Design review of the part built by this model. Coordinates are the model's own, in mm. Face numbers are marked on the shaded views. A direction names the side the tool comes from. Give positions to 0.01 mm unless a question says otherwise; leave off trailing zeros. Write each loop counter-clockwise with the first axis right and the second up, starting at its lowest first coordinate (ties: lowest second). Pieces come first, ordered by that corner, then holes. Notation, with made-up numbers: M 48,61 L 102,61 A22 cw 102,96 Z; hole C 82.25,-6.75 d8. An arc over 180 degrees is marked long. Answer in a Markdown table with one row per item.
```python
from build123d import *

# Parameters (mm, degrees)
F1_DEPTH = 15
F3_DEPTH = 54.4625242271
F5_DEPTH = 54.4625242271
F7_DEPTH = 53.9625242271
F8_R     = 5


with BuildPart() as f1:
    # F0 (on Top) → F1 (new body)
    with BuildSketch(Plane.XY):
        with BuildLine():
            Line((-25.9807621135, 15), (-30.3108891325, 17.5))
            ThreePointArc((-30.3108891325, 17.5), (-30.7987090687, 16.6264704522), (-31.2613615027, 15.7393544021))
            ThreePointArc((-31.2613615027, 15.7393544021), (-30.057560378, -17.9316219045), (-1, -34.9857113691))
            Line((-1, -34.9857113691), (-1, -32.5))
            Line((-1, -32.5), (1, -32.5))
            Line((1, -32.5), (1, -34.9857113691))
            ThreePointArc((1, -34.9857113691), (30.057560378, -17.9316219045), (31.2613615027, 15.7393544021))
            ThreePointArc((31.2613615027, 15.7393544021), (30.7987090687, 16.6264704522), (30.3108891325, 17.5))
            Line((30.3108891325, 17.5), (25.9807621135, 15))
            ThreePointArc((25.9807621135, 15), (0, -30), (-25.9807621135, 15))
        make_face()
        with BuildLine():
            ThreePointArc((-31.2613615027, 15.7393544021), (-30.7987090687, 16.6264704522), (-30.3108891325, 17.5))
            Line((-30.3108891325, 17.5), (-51.9615242271, 30))
            Line((-51.9615242271, 30), (-52.9615242271, 28.2679491924))
            Line((-52.9615242271, 28.2679491924), (-31.2613615027, 15.7393544021))
        make_face()
        with BuildLine():
            Line((-1, -32.5), (-1, -34.9857113691))
            ThreePointArc((-1, -34.9857113691), (0, -35), (1, -34.9857113691))
            Line((1, -34.9857113691), (1, -32.5))
            Line((1, -32.5), (-1, -32.5))
        make_face()
        with BuildLine():
            ThreePointArc((1, -34.9857113691), (0, -35), (-1, -34.9857113691))
            Line((-1, -34.9857113691), (-1, -57.5))
            Line((-1, -57.5), (1, -57.5))
            Line((1, -57.5), (1, -34.9857113691))
        make_face()
        with BuildLine():
            Line((51.9615242271, 30), (30.3108891325, 17.5))
            ThreePointArc((30.3108891325, 17.5), (30.7987090687, 16.6264704522), (31.2613615027, 15.7393544021))
            Line((31.2613615027, 15.7393544021), (52.9615242271, 28.2679491924))
            Line((52.9615242271, 28.2679491924), (51.9615242271, 30))
        make_face()
    extrude(amount=F1_DEPTH)

    # F2 (on face) → F3 (cut, through all)
    with BuildSketch(Plane(origin=(-1, -1.7320508076, 0), x_dir=(0.8660254038, -0.5, 0), z_dir=(-0.5, -0.8660254038, 0))):
        with BuildLine():
            Line((-37.4714052097, 15), (-57.4714052097, 15))
            ThreePointArc((-57.4714052097, 15), (-47.4714052097, 5), (-37.4714052097, 15))
        make_face()
    extrude(amount=-F3_DEPTH, mode=Mode.SUBTRACT)

    # F4 (on face) → F5 (cut, through all)
    with BuildSketch(Plane(origin=(1, -1.7320508076, 0), x_dir=(0.8660254038, 0.5, 0), z_dir=(0.5, -0.8660254038, 0))):
        with BuildLine():
            Line((57.4714052097, 15), (37.4714052097, 15))
            ThreePointArc((37.4714052097, 15), (47.4714052097, 5), (57.4714052097, 15))
        make_face()
    extrude(amount=-F5_DEPTH, mode=Mode.SUBTRACT)

    # F6 (on face) → F7 (cut, through all)
    with BuildSketch(Plane.YZ.offset(1)):
        with BuildLine():
            Line((-38.7428556845, 15), (-53.7428556845, 15))
            ThreePointArc((-53.7428556845, 15), (-46.2428556845, 7.5), (-38.7428556845, 15))
        make_face()
    extrude(amount=-F7_DEPTH, mode=Mode.SUBTRACT)

    # F8
    f8_edges = [f1.edges().sort_by_distance(p)[0] for p in [
        (-25.980762, 15, 7.5),
        (25.980762, 15, 7.5),
    ]]
    fillet(f8_edges, radius=F8_R)


solid = f1.part
```
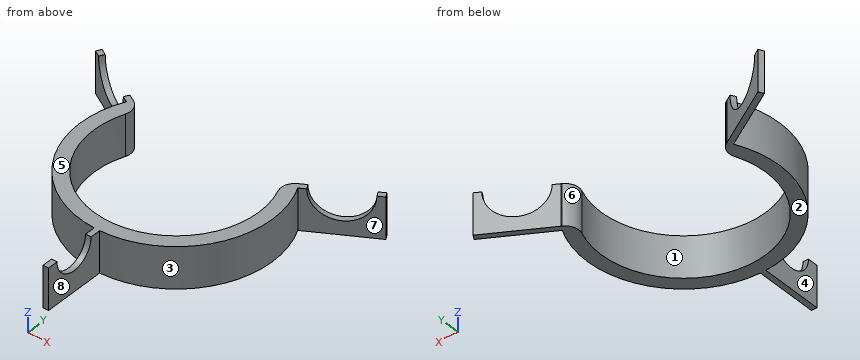
1) The part is to be moulded in two halves that separate along Y. For the marked faces 1, 2 and 3, say which applies: released by +Y, released by -Y, zero draft, split by the parting line, or undercut.
Geometry says:
| item | result |
|---|---|
| face 1 | undercut |
| face 2 | zero draft |
| face 3 | undercut |
2) Add section D-D (x = 17.5). Write out the cut boundary in (y, z), and give its area (3 significant figures).
Geometry says:
| item | result |
|---|---|
| outline | M -30.31,0 L -24.37,0 L -24.37,15 L -30.31,15 Z |
| area | 89.2 mm^2 |
3) Add section C-C (z = 3.25). Write out the cut boundary in (x, y).
Geometry says:
| item | result |
|---|---|
| outline | M -52.96,28.27 L -31.26,15.74 A35 ccw -1,-34.99 L -1,-57.5 L 1,-57.5 L 1,-34.99 A35 ccw 31.26,15.74 L 52.96,28.27 L 51.96,30 L 30,17.32 A5 ccw 27.86,11.13 A30 cw long -27.86,11.13 A5 ccw -30,17.32 L -51.96,30 Z |
4) To check wall thickness, follow probe 1 along X at (y, z) = (0, 11); probe 2 along Y at (x, z) = (0, 6.25); probe 3 along X at (y, z) = (-27, 4.5). State the ranges of each line that lie inside material, in increasing order. Write a range as [from, to].
Geometry says:
| item | result |
|---|---|
| probe 1 | [-35, -30], [30, 35] |
| probe 2 | [-57.5, -30] |
| probe 3 | [-22.27, -13.08], [13.08, 22.27] |
5) For the marked faces 4, 5, 6, 7 and 8, list the 3-axis set-ups (+Z, -Z, +X, -X, +Y, -Y) from which the entire face can be reached by the end or side of a thin tool; tool diameter is ignored.
Geometry says:
| item | result |
|---|---|
| face 4 | +Z, -Z, -X, -Y |
| face 5 | +Z, +X, -X, +Y, -Y |
| face 6 | +Z, -Z |
| face 7 | +Z, -Z, +X |
| face 8 | +Z, -Z, +X, -Y |
6) Add section B-B (z = 11.5). Write out the cut boundary in (x, y).
Geometry says:
| item | result |
|---|---|
| outline | M -52.96,28.27 L -50.22,26.69 L -49.22,28.42 L -51.96,30 Z; M -34,17.32 L -31.26,15.74 A35 ccw -1,-34.99 L -1,-39.61 L 1,-39.61 L 1,-34.99 A35 ccw 31.26,15.74 L 34,17.32 L 33,19.05 L 30,17.32 A5 ccw 27.86,11.13 A30 cw long -27.86,11.13 A5 ccw -30,17.32 L -33,19.05 Z; M -1,-57.5 L 1,-57.5 L 1,-52.88 L -1,-52.88 Z; M 49.22,28.42 L 50.22,26.69 L 52.96,28.27 L 51.96,30 Z |
7) Add section A-A (y = 0). Write out the cut boundary in (x, z), and give its area (3 significant figures).
Geometry says:
| item | result |
|---|---|
| outline | M -35,0 L -30,0 L -30,15 L -35,15 Z; M 30,0 L 35,0 L 35,15 L 30,15 Z |
| area | 150 mm^2 |
8) Insertion check: P1, Ø1.5, axis at x = 24.5, y = -27.5, coming from the -Z side; P2, Ø2, axis at x = 26.5, y = -17.5, coming from the -Z side; P3, Ø2, axis at y = -9, z = 7.5, coming from the +X side; P4, Ø1.5, axis at y = -9, z = 3.5, coming from the -X side. Each pin has a flat end and moves straight along its axis. Give the tip position at first contact, or say it passes through.
Geometry says:
| item | result |
|---|---|
| P1 | through |
| P2 | z = 0 |
| P3 | x = 34.07 |
| P4 | x = -34.01 |
